Design review of the part built by this model. Coordinates are the model's own, in mm. A direction names the side the tool comes from. Coordinates: 2 decimals unless noted, no trailing zeros. Order: outer loops, then holes, each group sorted by start corner. A loop starts at its lowest first (then second) coordinate and runs counter-clockwise, first axis right, second up. Notation, with made-up numbers: M -38,85.25 L -25,85.25 A22 ccw -25,114.25 Z; hole C 23,-10.5 d3. An arc over 180 degrees is marked long. Answer in a Markdown table with one row per item.
Autodesk Inventor part; units mm, degrees
ref_plane "YZ Plane" through (0, 0, 0) normal (1, 0, 0) x (0, 1, 0)
ref_plane "XZ Plane" through (0, 0, 0) normal (0, 1, 0) x (-1, 0, 0)
ref_plane "XY Plane" through (0, 0, 0) normal (0, 0, 1) x (1, 0, 0)
sketch "Sketch1" plane through (0, 0, 0) normal (0, 1, 0) x (-1, 0, 0)
  line L0 (0, 0) -> (40, 0)
  line L1 (40, 0) -> (40, -40)
  line L2 (40, -40) -> (0, -40)
  line L3 (0, -40) -> (0, 0)
  circle A0 centre (20, -20) radius 11.15
  dimension "d0" = 40
  dimension "d1" = 40
  dimension "d2" = 22.3
  dimension "d3" = 20
  dimension "d4" = 20
extrude "Extrusion1" add sketch "Sketch1" along normal blind 40
fillet "Fillet1" radius 12.7 2 edges at (0, 0, -20) (-40, 0, -20)
sketch "Sketch2" plane through (-40, 40, 0) normal (0, 0, 1) x (1, 0, 0)
  line L0 (8.85, -15) -> (31.15, -15)
  line L1 (31.15, -15) -> (31.15, -25)
  line L2 (31.15, -25) -> (8.85, -25)
  line L3 (8.85, -25) -> (8.85, -15)
  line L4 (8.85, -15) -> (31.15, -25) construction
  line L5 (31.15, -15) -> (8.85, -25) construction
  line L6 (40, -27.3) -> (40, 0)
  line L7 (27.3, -40) -> (12.7, -40)
  point P0 (40, -40)
  point P1 (20, -20)
  dimension "d8" = 20
  dimension "d9" = 22.3
  dimension "d10" = 10
  dimension "d11" = 15
extrude "Extrusion2" cut sketch "Sketch2" against normal blind 20
properties part number "YMountB"
(1) Draft analysis for pull direction X (two halves, no side actions). For faces 1 (the flat face through (-31.15, 20, -10)), 2 (the flat face through (0, 26, -20)), 3 (the cylindrical face through (-36.38, 3.82, -19.72)), 4 (the cylindrical face through (-18.548, 19.72, -31.055)), state which applies: pulls with the +X half, pulls with the -X half, needs draft (parallel to the pull), parting line crosses it, or undercut.
Return value:
| item | result |
|---|---|
| face 1 | undercut |
| face 2 | pulls with the +X half |
| face 3 | pulls with the -X half |
| face 4 | undercut |
(2) For line 1 along X through (y, z) = (23, -20); line 2 along Y through (x, z) = (-18, -2.5), list the stretches that pass through material, from the lowest coordinate up. Write a range as from..to.
Return value:
| item | result |
|---|---|
| line 1 | x = -40..-31.15, -8.85..0 |
| line 2 | y = 0..15, 25..40 |
(3) Add section A-A, the plane x = -20. Give the boundary of the cut face in (y, z), and give its area (4 significant figures).
Return value:
| item | result |
|---|---|
| outline | M 0,-40 L 40,-40 L 40,-31.15 L 0,-31.15 Z; M 0,-8.85 L 15,-8.85 L 15,0 L 0,0 Z; M 25,-8.85 L 40,-8.85 L 40,0 L 25,0 Z |
| area | 619.5 mm2 |
(4) Add section B-B, the plane z = -13.5. Give the boundary of the cut face in (x, y), and give its area (3 significant figures).
Return value:
| item | result |
|---|---|
| outline | M -40,12.7 A12.7 ccw -29.06,0.12 L -29.06,15 L -31.15,15 L -31.15,25 L -29.06,25 L -29.06,40 L -40,40 Z; M -10.94,0.12 A12.7 ccw 0,12.7 L 0,40 L -10.94,40 L -10.94,25 L -8.85,25 L -8.85,15 L -10.94,15 Z |
| area | 764 mm2 |
(5) Insertion check: pin 1 Ø10 at (y, z) = (4.5, -29.5) entering from -X; pin 2 Ø1 at (y, z) = (8.5, -12.5) entering from -X. Each pin has a flat end and moves straight along its axis. Give the tip position at first contact, or say it passes through.
Return value:
| item | result |
|---|---|
| pin 1 | stops at x = -39.59 |
| pin 2 | stops at x = -39.45 |
(6) Add section D-D, the plane z = -32.5. Give the boundary of the cut face in (x, y), and give its area (3 significant figures).
Return value:
| item | result |
|---|---|
| outline | M -40,12.7 A12.7 ccw -27.3,0 L -12.7,0 A12.7 ccw 0,12.7 L 0,40 L -40,40 Z |
| area | 1,530 mm2 |
(7) Add section C-C, the plane y = 24. Give the boundary of the cut face in (x, z), and give its area (3 significant figures).
Return value:
| item | result |
|---|---|
| outline | M -40,-40 L 0,-40 L 0,0 L -8.85,0 L -8.85,-20 A11.15 cw -31.15,-20 L -31.15,0 L -40,0 Z |
| area | 959 mm2 |
(8) For faces 5 (the flat face through (-11, 40, -11)), 6 (the flat face through (-20, 25, -5)), list the 3-axis set-ups (+Z, -Z, +X, -X, +Y, -Y) from which the entire face can be reached by the end or side of a thin tool; tool diameter is ignored.
Return value:
| item | result |
|---|---|
| face 5 | +Z, -Z, +X, -X, +Y |
| face 6 | +Z |
